Input: part model. Units: mm. Frame: model coordinates. Face numbers are marked on the shaded views. A direction names the side the tool comes from. Coordinates: 2 decimals unless noted, no trailing zeros. Order: outer loops, then holes, each group sorted by start corner. A loop starts at its lowest first (then second) coordinate and runs counter-clockwise, first axis right, second up.
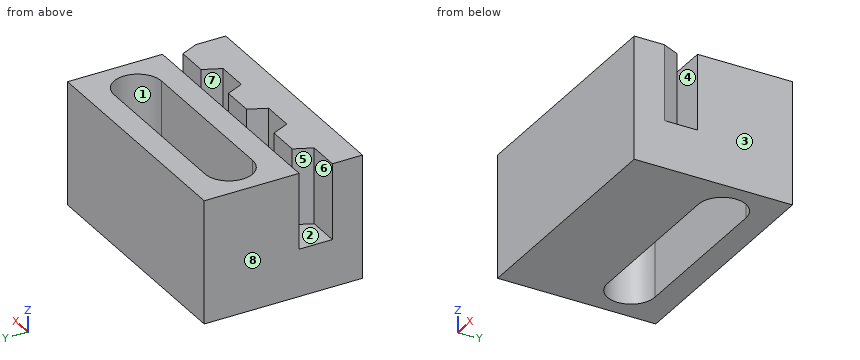
from build123d import *

# Parameters (mm, degrees)
F0_W     = 15
F0_H     = 10
F1_DEPTH = 3
F2_W     = 15
F2_H     = 6
F3_DEPTH = 4.8
F5_DEPTH = 7.801


with BuildPart() as f1:
    # F0 (on Top) → F1 (new body)
    with BuildSketch(Plane.XY):
        Rectangle(F0_W, F0_H)
    extrude(amount=F1_DEPTH)

    # F2 (on face) → F3 (join)
    with BuildSketch(Plane.XY.offset(3)):
        Polygon((2, -2), (0, -2), (-0.5, -3.1), (-2.5, -3.1), (-3, -2), (-5, -2), (-5.5, -3.1), (-7.5, -3.1), (-7.5, -5), (7.5, -5), (7.5, -3.1), (7, -2), (5, -2), (4.5, -3.1), (2.5, -3.1), align=None)
        with Locations((0, 2)):
            Rectangle(F2_W, F2_H)
    extrude(amount=F3_DEPTH)

    # F4 (on face) → F5 (cut, through all)
    with BuildSketch(Plane.XY.offset(7.8)):
        with BuildLine():
            Line((5, 3.5), (-5, 3.5))
            ThreePointArc((-5, 3.5), (-6.5, 2), (-5, 0.5))
            Line((-5, 0.5), (5, 0.5))
            ThreePointArc((5, 0.5), (6.5, 2), (5, 3.5))
        make_face()
    extrude(amount=-F5_DEPTH, mode=Mode.SUBTRACT)


solid = f1.part
Item 1: Ray query, probe 1 along Y at (x, z) = (-0.75, 6.25); probe 2 along Y at (x, z) = (1.5, 5); probe 3 along Y at (x, z) = (1, 2.5). Return the intervals inside material, ascending.
Response values:
probe 1: y = -5 to -3.1, -1 to 0.5, 3.5 to 5
probe 2: y = -5 to -2, -1 to 0.5, 3.5 to 5
probe 3: y = -5 to 0.5, 3.5 to 5
Item 2: Pin query (flat end, axial travel): pin 1 Ø3 at (x, y) = (5.5, 2) entering from +Z. Return the tip coordinate at first contact, or that it passes through.
Response values:
pin 1: stops at z = 7.8
Item 3: Cut plane B-B on z = 0.75. Return loops of the section in (x, y).
Response values:
outline: (-7.5, -5) - (7.5, -5) - (7.5, 5) - (-7.5, 5) - close; hole (-5, 0.5) - (5, 0.5) arc R1.5 ccw to (5, 3.5) - (-5, 3.5) arc R1.5 ccw to start
Item 4: Draft query along X for the marked faces 6, 7 and 8. Return one class per face: pulls with the +X half, pulls with the -X half, needs draft (parallel to the pull), parting line crosses it, or undercut.
Response values:
face 6: needs draft
face 7: undercut
face 8: pulls with the -X half
Item 5: Access query for the marked faces 1, 2, 3, 4 and 5. Directions: +Z, -Z, +X, -X, +Y, -Y. A direction counts if a zero-diameter tool reaches every point of the face in a straight line with its end or side. Return the directions, or none.
Response values:
face 1: +Z, -Z
face 2: +Z
face 3: +Z, -Z, +X, +Y, -Y
face 4: +Z, +X, -X
face 5: +Z, -X
Item 6: Cut plane D-D on y = 2. Return loops of the section in (x, z), then the cut area to 3 significant figures.
Response values:
outline: (-7.5, 0) - (-6.5, 0) - (-6.5, 7.8) - (-7.5, 7.8) - close; (6.5, 0) - (7.5, 0) - (7.5, 7.8) - (6.5, 7.8) - close
area: 15.6 mm2
Item 7: Cut plane C-C on z = 4.25. Return loops of the section in (x, y), then the cut area to 3 significant figures.
Response values:
outline: (-7.5, -5) - (7.5, -5) - (7.5, -3.1) - (7, -2) - (5, -2) - (4.5, -3.1) - (2.5, -3.1) - (2, -2) - (0, -2) - (-0.5, -3.1) - (-2.5, -3.1) - (-3, -2) - (-5, -2) - (-5.5, -3.1) - (-7.5, -3.1) - close; (-7.5, -1) - (7.5, -1) - (7.5, 5) - (-7.5, 5) - close; hole (-5, 0.5) - (5, 0.5) arc R1.5 ccw to (5, 3.5) - (-5, 3.5) arc R1.5 ccw to start
area: 89.7 mm2
Item 8: Cut plane A-A on x = -1. Return loops of the section in (y, z), then the cut area to 3 significant figures.
Response values:
outline: (-5, 0) - (0.5, 0) - (0.5, 7.8) - (-1, 7.8) - (-1, 3) - (-3.1, 3) - (-3.1, 7.8) - (-5, 7.8) - close; (3.5, 0) - (5, 0) - (5, 7.8) - (3.5, 7.8) - close
area: 44.5 mm2
